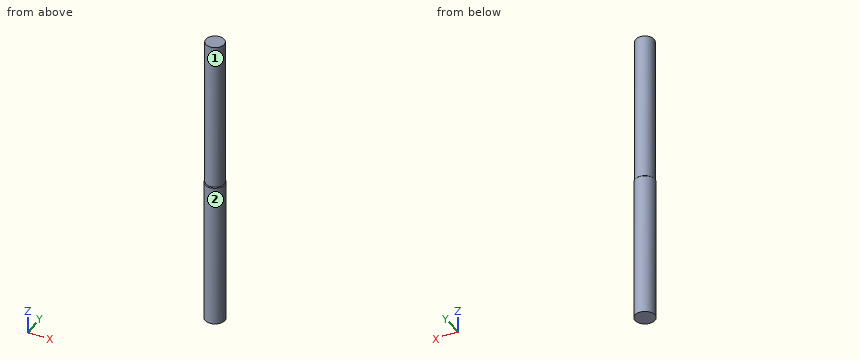
```python
from build123d import *

# Parameters (mm, degrees)
F0_R        = 5.08
F1_DEPTH    = 76.2
F2_R        = 4.699
F3_DEPTH    = 76.2
F4_S5_R     = 4.699
F4_T6_DEPTH = 9


# Not quite as in the source:
# - a fillet or chamfer that OpenCascade refuses, or shapes differently, is made with other operations: its cross-section is extruded or revolved along the edge and cut away or added


with BuildPart() as f1:
    # F0 (on Top) → F1 (new body)
    with BuildSketch(Plane.XY):
        Circle(F0_R)
    extrude(amount=-F1_DEPTH)

    # F2 (on face) → F3 (join)
    with BuildSketch(Plane.XY):
        Circle(F2_R)
    extrude(amount=F3_DEPTH)

    # F4: chamfer of 1.27 on 1 edges, made by hand


with BuildPart() as f4_tool2:
    # F4_s3 → F4_t4 (revolve)
    with BuildSketch(Plane.XZ):
        Polygon((5.08, -1.27), (3.81, 0), (5.08, 0), align=None)
    revolve(axis=Axis((0, 0, 0), (0, 0, 1)))

    # F4_s5 → F4_t6 (cut, symmetric)
    with BuildSketch(Plane.XY.offset(-0.6)):
        Circle(F4_S5_R)
    extrude(amount=F4_T6_DEPTH, both=True, mode=Mode.SUBTRACT)


with BuildPart() as f1_1:
    add(f1.part)

    # F4_t1: cut F4_tool2
    add(f4_tool2.part, mode=Mode.SUBTRACT)


solid = f1_1.part
```
Source: CAD feature listing. Evaluate the final solid. Frame: model axes, mm. Face numbers are marked on the shaded views. A direction names the side the tool comes from. Round coordinates to 2 decimals unless told otherwise and drop trailing zeros. Loops run counter-clockwise (first coordinate to the right, second up) from the corner with the lowest first, then second, coordinate; pieces in that order, holes last. Notation, with made-up numbers: M 33,57.5 L 74,57.5 A19 cw 74,89.5 Z; hole C 6.25,42.25 d2. An arc over 180 degrees is marked long. Use a Markdown table: item, result. Add a question column.
1. Reachability of the marked faces 1 and 2 from +Z, -Z, +X, -X, +Y, -Y: full face, straight path, thin tool, end or side. Return the list, or none.
2. Section query C-C on z = 55. Return the cut outline in (x, y), then the cut area to 3 significant figures.
3. Section query A-A on y = 0. Return the cut outline in (x, z).
4. Line query: line 1 (X direction, y = -2, z = -58); line 2 (X direction, y = -4, z = 21); line 3 (Y direction, x = 1, z = 47.5). Output: solid intervals per line, ascending.
Reported:
| question | item | result |
|---|---|---|
| 1 | face 1 | +Z |
| 1 | face 2 | +Z, -Z |
| 2 | outline | C 0,0 d9.4 |
| 2 | area | 69.4 mm² |
| 3 | outline | M -5.08,-76.2 L 5.08,-76.2 L 5.08,-1.27 L 4.7,-0.89 L 4.7,76.2 L -4.7,76.2 L -4.7,-0.89 L -5.08,-1.27 Z |
| 4 | line 1 | x = -4.67 to 4.67 |
| 4 | line 2 | x = -2.47 to 2.47 |
| 4 | line 3 | y = -4.59 to 4.59 |
